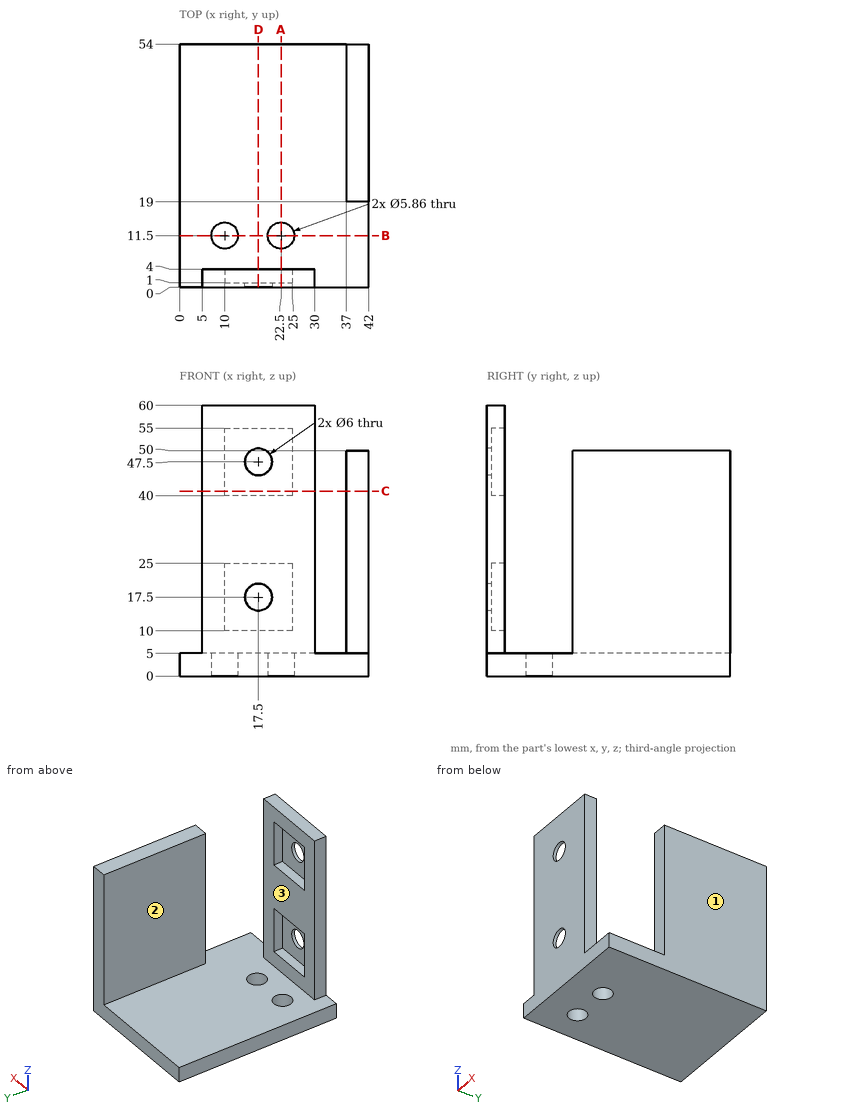
Study the drawing (mm; zero at the part's minimum x, y, z) and answer. A direction names the side the tool comes from. Round coordinates to 2 decimals unless told otherwise and drop trailing zeros. Write each loop counter-clockwise with the first axis right and the second up, starting at its lowest first coordinate (ties: lowest second). Pieces come first, ordered by that corner, then holes. Notation, with made-up numbers: (45, -13) - (102, -13) arc R21 ccw to (102, -6) - close; hole circle Ø9 at (-38, 52). An arc over 180 degrees is marked (long way). Use a Markdown table: item, result. Add a question column.
1. The part is cut by section A-A (x = 22.5). Write down the section's boundary in (y, z), and give its area (3 significant figures).
2. The part is cut by section B-B (y = 11.5). Write down the section's boundary in (x, z), and give its area (3 significant figures).
3. Consider line 1 (X direction, y = 11.5, z = 3.05); line 2 (Z direction, x = 17.5, y = 0.25); line 3 (Z direction, x = 17, y = 41.5). Determine where each line is inside the solid, lowest interval first.
4. The part is cut by section D-D (x = 17.5). Write down the section's boundary in (y, z), and give its area (3 significant figures).
5. Flat-ended cylindrical pins translate along their axes: P1, Ø1, axis at x = 16, y = 39, coming from the +Z side; P2, Ø20, axis at x = 17, z = 28.5, coming from the +Y side; P3, Ø5.5, axis at x = 22.5, y = 11.5, coming from the -Z side; P4, Ø4.5, axis at x = 16, z = 17.5, coming from the +Y side. Find the tip coordinate at first contact, or state that the pin passes through.
6. A tool of negligible diameter and unlimited length cuts with its end or side. For the marked faces 1, 2 and 3, from which of +Z, -Z, +X, -X, +Y, -Y can it reach the whole face along a straight path? Write none if from no direction.
7. The part is cut by section C-C (z = 41). Write down the section's boundary in (x, y).
Reported:
| question | item | result |
|---|---|---|
| 1 | outline | (0, 0) - (8.57, 0) - (8.57, 5) - (4, 5) - (4, 10) - (1, 10) - (1, 25) - (4, 25) - (4, 40) - (1, 40) - (1, 55) - (4, 55) - (4, 60) - (0, 60) - close; (14.43, 0) - (54, 0) - (54, 5) - (14.43, 5) - close |
| 1 | area | 371 mm^2 |
| 2 | outline | (0, 0) - (7.07, 0) - (7.07, 5) - (0, 5) - close; (12.93, 0) - (19.57, 0) - (19.57, 5) - (12.93, 5) - close; (25.43, 0) - (42, 0) - (42, 5) - (25.43, 5) - close |
| 2 | area | 151 mm^2 |
| 3 | line 1 | 0 to 7.07, 12.93 to 19.57, 25.43 to 42 |
| 3 | line 2 | 0 to 14.5, 20.5 to 44.5, 50.5 to 60 |
| 3 | line 3 | 0 to 5 |
| 4 | outline | (0, 0) - (54, 0) - (54, 5) - (4, 5) - (4, 10) - (1, 10) - (1, 14.5) - (0, 14.5) - close; (0, 20.5) - (1, 20.5) - (1, 25) - (4, 25) - (4, 40) - (1, 40) - (1, 44.5) - (0, 44.5) - close; (0, 50.5) - (1, 50.5) - (1, 55) - (4, 55) - (4, 60) - (0, 60) - close |
| 4 | area | 388 mm^2 |
| 5 | P1 | z = 5 |
| 5 | P2 | y = 4 |
| 5 | P3 | through |
| 5 | P4 | y = 1 |
| 6 | face 1 | +Z, -Z, +X, +Y, -Y |
| 6 | face 2 | +Z, -X, +Y, -Y |
| 6 | face 3 | +Z, +X, -X, +Y |
| 7 | outline | (5, 0) - (30, 0) - (30, 4) - (25, 4) - (25, 1) - (10, 1) - (10, 4) - (5, 4) - close; (37, 19) - (42, 19) - (42, 54) - (37, 54) - close |
